The drawing under review shows one solid part. Ordinate dimensions are in mm from its lowest x, y, z. Round coordinates to 2 decimals unless told otherwise and drop trailing zeros. Order: outer loops, then holes, each group sorted by start corner. A loop starts at its lowest first (then second) coordinate and runs counter-clockwise, first axis right, second up. Notation, with made-up numbers: M 33,23.25 L 60,23.25 A20 ccw 60,55.25 Z; hole C 11.25,44.5 d6. An arc over 180 degrees is marked long. Answer as a JSON object with one key per item and string values. Group by question number.
1) Consider section A-A, the plane z = 10. Write out the cut boundary in (x, y), then the cut area to 3 significant figures.
2) Consider section C-C, the plane x = 16.5. Write out the cut boundary in (y, z).
3) To check wall thickness, follow line 1 (Y direction, x = 51.5, z = 10); line 2 (Y direction, x = 13, z = 12.75) (1 decimal). State the ranges of each line that lie inside material, in increasing order.
4) Consider section B-B, the plane y = 44. Write out the cut boundary in (x, z).
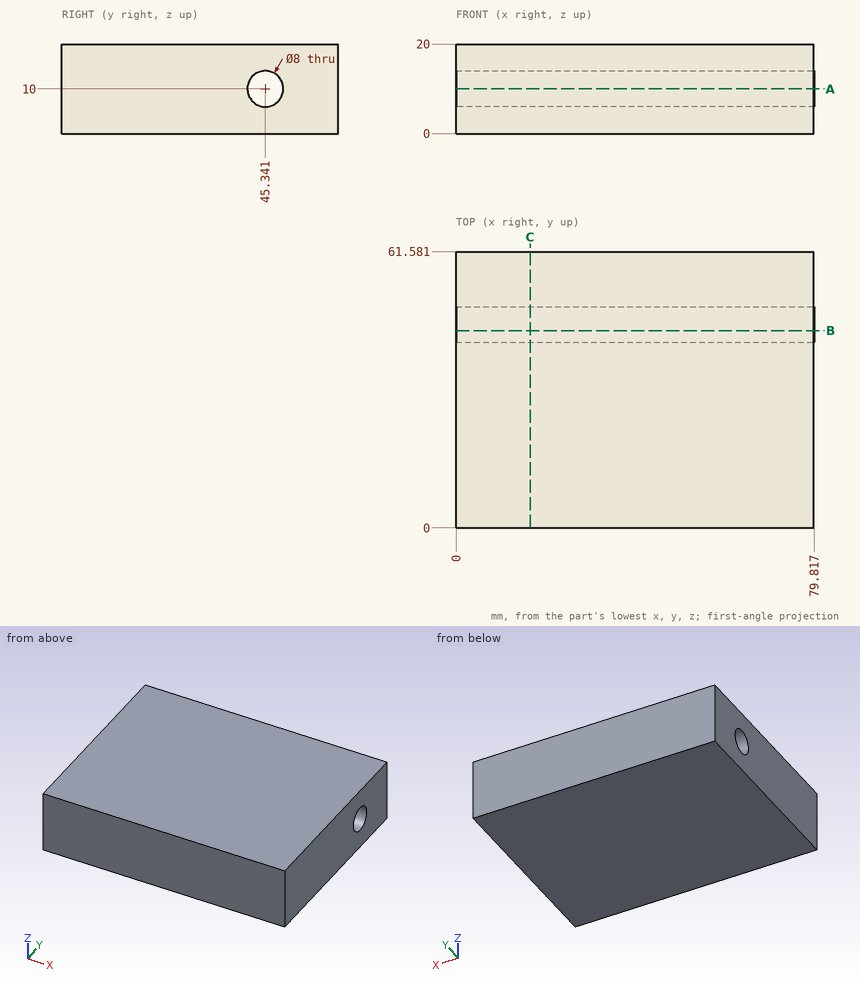
Results list:
{
 "1": {"outline": "M 0,0 L 79.82,0 L 79.82,41.34 L 0,41.34 Z; M 0,49.34 L 79.82,49.34 L 79.82,61.58 L 0,61.58 Z", "area": "4,280 mm^2"},
 "2": {"outline": "M 0,0 L 61.58,0 L 61.58,20 L 0,20 Z; hole C 45.34,10 d8"},
 "3": {"line 1": "0 to 41.34, 49.34 to 61.58", "line 2": "0 to 42.4, 48.2 to 61.6"},
 "4": {"outline": "M 0,0 L 79.82,0 L 79.82,6.23 L 0,6.23 Z; M 0,13.77 L 79.82,13.77 L 79.82,20 L 0,20 Z"}
}
